Geometry: final body of the model. Coordinates: model frame, mm. A direction names the side the tool comes from. Coordinates: 2 decimals unless noted, no trailing zeros. Write each loop counter-clockwise with the first axis right and the second up, starting at its lowest first coordinate (ties: lowest second). Pieces come first, ordered by that corner, then holes. Notation, with made-up numbers: (-26, 71) -> (9, 71) arc R22 ccw to (9, 96) -> close; hole circle Ø1 at (53, 61). An arc over 180 degrees is marked (long way). One line per item, written item: value.
Autodesk Inventor part; units mm, degrees
ref_plane "YZ Plane" through (0, 0, 0) normal (1, 0, 0) x (0, 1, 0)
ref_plane "XZ Plane" through (0, 0, 0) normal (0, 1, 0) x (-1, 0, 0)
ref_plane "XY Plane" through (0, 0, 0) normal (0, 0, 1) x (1, 0, 0)
sketch "Sketch1" plane through (0, 0, 0) normal (0, 0, 1) x (1, 0, 0)
  line L0 (-7.5, 6) -> (7.5, 6)
  line L1 (7.5, 6) -> (7.5, 0)
  line L2 (7.5, 0) -> (-7.5, 0)
  line L3 (-7.5, 0) -> (-7.5, 6)
  line L4 (-7.5, 6) -> (7.5, 0) construction
  line L5 (7.5, 6) -> (-7.5, 0) construction
  line L6 (-16, 12) -> (16, 12)
  line L7 (16, 12) -> (16, 0)
  line L8 (16, 0) -> (-16, 0)
  line L9 (-16, 0) -> (-16, 12)
  line L10 (-16, 12) -> (16, 0) construction
  line L11 (16, 12) -> (-16, 0) construction
  point P0 (0, 0)
  point P1 (0, 3)
  point P2 (0, 0)
  point P3 (0, 6)
  point P4 (7.5, 0)
  point P5 (-7.5, 0)
  dimension "d0" = 15
  dimension "d1" = 6
  dimension "d2" = 32
  dimension "d3" = 12
extrude "Extrusion1" add sketch "Sketch1" along normal mid plane 42.1 contours L3 L8 L9 L6 L7 L1 L0
sketch "Sketch2" plane through (-16, 12, 21.05) normal (0, 1, 0) x (1, 0, 0)
  line L0 (28.5, 11.05) -> (3.5, 11.05) construction
  line L1 (3.5, 11.05) -> (3.5, 31.05) construction
  line L2 (3.5, 31.05) -> (28.5, 31.05) construction
  line L3 (28.5, 31.05) -> (28.5, 11.05) construction
  line L4 (28.5, 11.05) -> (3.5, 31.05) construction
  line L5 (3.5, 11.05) -> (28.5, 31.05) construction
  point P0 (16, 21.05)
  dimension "d6" = 25
  dimension "d7" = 20
hole "Hole1" at (-12.5, 12, 10) at (12.5, 12, 10) at (12.5, 12, -10) at (-12.5, 12, -10) direction (0, -1, 0) diameter 2.459 depth 4
fillet "Fillet1" radius 1 4 edges at (16, 12, 0) (-16, 12, 0) (16, 0, 0) (-16, 0, 0)
properties part number "MGN12C Cart" material "Steel, Carbon"
(1) Section D-D (z = 3). Return the cut outline in (x, y), then the cut area to 3 significant figures.
Responses:
outline: (-16, 1) arc R1 ccw to (-15, 0) -> (-7.5, 0) -> (-7.5, 6) -> (7.5, 6) -> (7.5, 0) -> (15, 0) arc R1 ccw to (16, 1) -> (16, 11) arc R1 ccw to (15, 12) -> (-15, 12) arc R1 ccw to (-16, 11) -> close
area: 293 mm2
(2) Pull-direction query (Z, two-part tool) for faces 1 (the cylindrical face through (-12.869, 9.972, 11.173)), 2 (the cylindrical face through (15.699, 11.715, -0.295)), 3 (the cylindrical face through (12.131, 9.972, 11.173)); classes: released by +Z, released by -Z, zero draft, split by the parting line, or undercut.
Responses:
face 1: undercut
face 2: zero draft
face 3: undercut
(3) Line query: line 1 (Z direction, x = 12.5, y = 10.85); line 2 (X direction, y = 8.9, z = -10); line 3 (X direction, y = 4.5, z = 4). Output: solid intervals per line, ascending. Write a range as [from, to].
Responses:
line 1: z = [-21.05, -11.23], [-8.77, 8.77], [11.23, 21.05]
line 2: x = [-16, -13.73], [-11.27, 11.27], [13.73, 16]
line 3: x = [-16, -7.5], [7.5, 16]
(4) Section A-A (y = 2.5). Return the cut outline in (x, z), then the cut area to 3 significant figures.
Responses:
outline: (-16, -21.05) -> (-7.5, -21.05) -> (-7.5, 21.05) -> (-16, 21.05) -> close; (7.5, -21.05) -> (16, -21.05) -> (16, 21.05) -> (7.5, 21.05) -> close
area: 716 mm2
(5) First-contact query: pin 1 (0.7 mm diameter, centred on x = -12.5, z = -10, fed in from +Y); pin 2 (4.5 mm diameter, centred on x = 1.5, z = 6.5, fed in from -Y). Flat tips, straight axial feed; report the tip coordinate or a pass-through.
Responses:
pin 1: stops at y = 8
pin 2: stops at y = 6
(6) Section B-B (x = 12.5). Return the cut outline in (y, z).
Responses:
outline: (0, -21.05) -> (12, -21.05) -> (12, -11.23) -> (8, -11.23) -> (8, -8.77) -> (12, -8.77) -> (12, 8.77) -> (8, 8.77) -> (8, 11.23) -> (12, 11.23) -> (12, 21.05) -> (0, 21.05) -> close
(7) Section C-C (z = -10). Return the cut outline in (x, y).
Responses:
outline: (-16, 1) arc R1 ccw to (-15, 0) -> (-7.5, 0) -> (-7.5, 6) -> (7.5, 6) -> (7.5, 0) -> (15, 0) arc R1 ccw to (16, 1) -> (16, 11) arc R1 ccw to (15, 12) -> (13.73, 12) -> (13.73, 8) -> (11.27, 8) -> (11.27, 12) -> (-11.27, 12) -> (-11.27, 8) -> (-13.73, 8) -> (-13.73, 12) -> (-15, 12) arc R1 ccw to (-16, 11) -> close
(8) Reachability of faces 4 (the cylindrical face through (-12.869, 9.972, -8.827)), 5 (the flat face through (-7.5, 3, 0)), 6 (the cylindrical face through (15.715, 0.301, -0.295)) from +Z, -Z, +X, -X, +Y, -Y: full face, straight path, thin tool, end or side. Return the list, or none.
Responses:
face 4: +Y
face 5: +Z, -Z, -Y
face 6: +Z, -Z, +X, -Y
